Design review of the part shown in the three views and the two pictorial views. Dimensions are in mm from the part's minimum x, y and z. Round coordinates to 2 decimals unless told otherwise and drop trailing zeros. Write each loop counter-clockwise with the first axis right and the second up, starting at its lowest first coordinate (ties: lowest second). Pieces come first, ordered by that corner, then holes. Notation, with made-up numbers: (69.5, 83) - (107.5, 83) arc R7 ccw to (107.5, 89) - close; hole circle Ø6 at (87, 21). An arc over 180 degrees is marked (long way). Use one line per item in the form item = value.
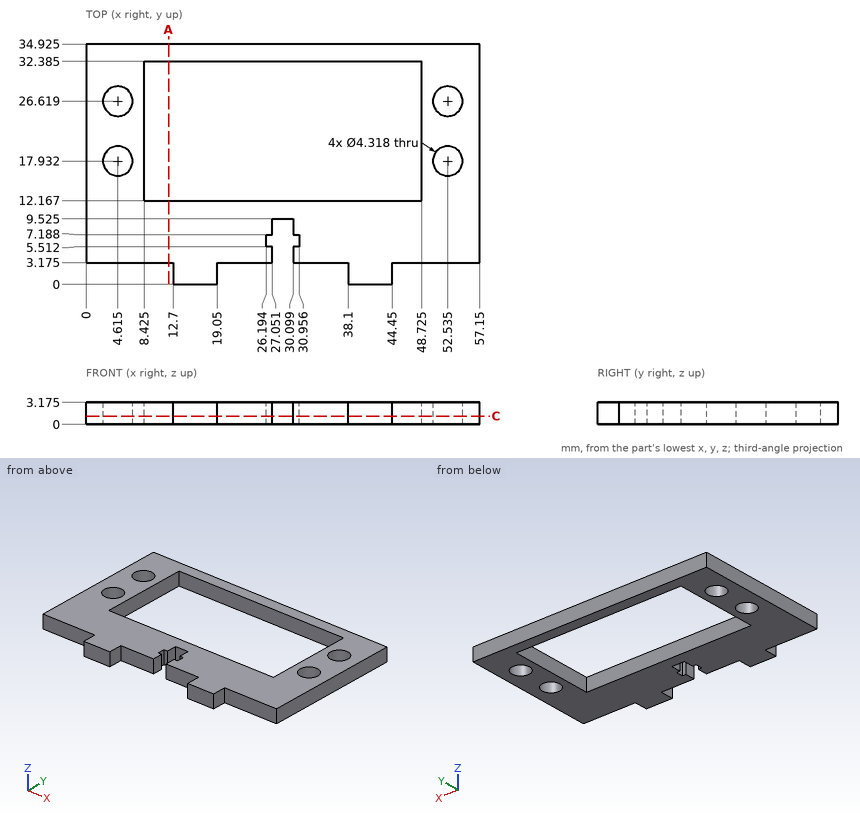
Q1. We need section A-A on x = 12. Write out the cut boundary in (y, z) (1 decimal).
Calculated:
outline = (3.2, 0) - (12.2, 0) - (12.2, 3.2) - (3.2, 3.2) - close; (32.4, 0) - (34.9, 0) - (34.9, 3.2) - (32.4, 3.2) - close
Q2. We need section C-C on z = 1.2. State how many separate pieces and enclosed holes the cut face has.
Calculated:
separate_pieces = 1
enclosed_holes = 5
Q3. For P1, Ø4, axis at x = 52.54, y = 26.62, coming from the -Z side; P2, Ø1, axis at y = 1, z = 2, coming from the -X side; P3, Ø1.6, axis at x = 50.5, z = 1.5, coming from the -Y side (3 decimals); P4, Ø0.9, axis at x = 29, z = 1.5, coming from the -Y side (3 decimals), all flat-tipped, find the tip position at first contact; note any pin that passes through.
Calculated:
P1 = through
P2 = 12.7
P3 = 3.175
P4 = 9.525
Q4. To check wall thickness, follow line 1 along Y through (x, z) = (4.5, 0.8) (1 decimal); line 2 along Y through (x, z) = (42.5, 2) (1 decimal); line 3 along Y through (x, z) = (48.5, 0.65) (1 decimal). State the ranges of each line that lie inside material, in increasing order. Write a range as from..to.
Calculated:
line_1 = 3.2..15.8, 20.1..24.5, 28.8..34.9
line_2 = 0..12.2, 32.4..34.9
line_3 = 3.2..12.2, 32.4..34.9
